```python
from build123d import *

# Parameters (mm, degrees)
SKETCH1_R           = 3
SKETCH1_R_2         = 1.6
BOSS_EXTRUDE1_DEPTH = 2.2
SKETCH1_3_R         = 1.6
BOSS_EXTRUDE2_DEPTH = 1
SKETCH5_R           = 1.5
BOSS_EXTRUDE3_DEPTH = 1
SKETCH6_R           = 2
BOSS_EXTRUDE4_DEPTH = 1
SKETCH8_R           = 1.5
BOSS_EXTRUDE5_DEPTH = 3
SKETCH10_R          = 2
BOSS_EXTRUDE6_DEPTH = 1


with BuildPart() as part:
    # Sketch1 → Boss-Extrude1 (new body)
    with BuildSketch(Plane(origin=(0, 0, 0), x_dir=(1, 0, 0), z_dir=(0, 1, 0))):
        with Locations((-0.522013312, 0.511138034)):
            Circle(SKETCH1_R)
        with Locations((-0.522013312, 0.511138034)):
            Circle(SKETCH1_R_2, mode=Mode.SUBTRACT)
    extrude(amount=BOSS_EXTRUDE1_DEPTH)

    # Sketch1_3 → Boss-Extrude2 (add)
    with BuildSketch(Plane(origin=(0, 0, 0), x_dir=(1, 0, 0), z_dir=(0, 1, 0))):
        with Locations((-0.522013312, 0.511138034)):
            Circle(SKETCH1_3_R)
    extrude(amount=BOSS_EXTRUDE2_DEPTH)

    # Sketch5 → Boss-Extrude3 (add)
    with BuildSketch(Plane.XZ):
        with Locations((-0.522013312, -0.511138034)):
            Circle(SKETCH5_R)
    extrude(amount=BOSS_EXTRUDE3_DEPTH)

    # Sketch6 → Boss-Extrude4 (add)
    with BuildSketch(Plane.XZ.offset(1)):
        with Locations((-0.522013312, -0.511138034)):
            Circle(SKETCH6_R)
    extrude(amount=BOSS_EXTRUDE4_DEPTH)

    # Sketch8 → Boss-Extrude5 (add)
    with BuildSketch(Plane(origin=(0, -2, 0), x_dir=(-1, 0, 0), z_dir=(0, -1, 0))):
        with Locations((0.522013312, 0.511138034)):
            Circle(SKETCH8_R)
    extrude(amount=BOSS_EXTRUDE5_DEPTH)

    # Sketch10 → Boss-Extrude6 (add)
    with BuildSketch(Plane.XZ.offset(5)):
        with Locations((-0.522013312, -0.511138034)):
            Circle(SKETCH10_R)
    extrude(amount=-BOSS_EXTRUDE6_DEPTH)


solid = part.part
```
Verification items for the finished model (mm, model axes). A direction names the side the tool comes from. Coordinates: 2 decimals unless noted, no trailing zeros. Write each loop counter-clockwise with the first axis right and the second up, starting at its lowest first coordinate (ties: lowest second). Pieces come first, ordered by that corner, then holes. Notation, with made-up numbers: M 89.5,5 L 141.5,5 A24 cw 141.5,34 Z; hole C 72,27.5 d6. An arc over 180 degrees is marked long. Answer as a JSON object with one key per item and string values. Group by question number.
(1) Cross-section at A-A, the plane z = 1.3. Record the cut outline in (x, y), and give its area (3 significant figures).
(2) Tool access check on faces 1 (the face through (-1, 1, -1)), 2 (the face through (0.91, -0.49, -0.06)), 3 (the face through (1.325, -1.493, -1.277)). Record the directions out of +Z, -Z, +X, -X, +Y, -Y that give a thin tool (end or side, any length) a straight path to the whole face; none if there is none.
(3) Gauge pin test, flat ends, axial feed: pin 1 (1.5 mm diameter, centred on y = -1.5, z = 0.5, fed in from -X); pin 2 (1.5 mm diameter, centred on x = -2, z = -0.5, fed in from +Y); pin 3 (1.5 mm diameter, centred on x = 1.5, z = 2, fed in from -Y); pin 4 (1 mm diameter, centred on x = 0, z = -1, fed in from +Y). Record the tip position at first contact, or that the pin passes through.
(4) Material ranges on line 1 (Y direction, x = -0.8, z = -0.15); line 2 (Z direction, x = -0.5, y = 1.75); line 3 (Y direction, x = -3.15, z = -1), recorded low to high.
(5) Cross-section at C-C, the plane z = 0.2. Record the cut outline in (x, y), and give its area (3 significant figures).
(6) Cross-section at B-B, the plane x = -2.4. Record the cut outline in (y, z).
(7) Release check for a two-part mould opening along X. For faces 4 (the face through (1, 0, 1)), 5 (the face through (-0.197, -2.986, 0.953)), 6 (the face through (1, 2, -1)) record: +X half, -X half, draft (parallel to the pull), parting line (faces both ways), or undercut.
(8) Cross-section at D-D, the plane x = 0.8. Record the cut outline in (y, z), and give its area (3 significant figures).
Reply:
{
 "1": {"outline": "M -2.91,0 L 1.87,0 L 1.87,2.2 L -2.91,2.2 Z; M -1.37,-5 L 0.33,-5 L 0.33,-4 L -1.37,-4 Z; M -1.37,-2 L 0.33,-2 L 0.33,-1 L -1.37,-1 Z", "area": "13.9 mm²"},
 "2": {"face 1": "+Y", "face 2": "none", "face 3": "-Y"},
 "3": {"pin 1": "x = -2.5", "pin 2": "y = 2.2", "pin 3": "y = 0", "pin 4": "y = 1"},
 "4": {"line 1": "-5 to 1", "line 2": "-3.51 to -2.11, 1.09 to 2.49", "line 3": "0 to 2.2"},
 "5": {"outline": "M -3.44,0 L -1.84,0 L -1.84,-1 L -2.39,-1 L -2.39,-2 L -1.84,-2 L -1.84,-4 L -2.39,-4 L -2.39,-5 L 1.35,-5 L 1.35,-4 L 0.8,-4 L 0.8,-2 L 1.35,-2 L 1.35,-1 L 0.8,-1 L 0.8,0 L 2.39,0 L 2.39,2.2 L 0.91,2.2 L 0.91,1 L -1.96,1 L -1.96,2.2 L -3.44,2.2 Z", "area": "24.8 mm²"},
 "6": {"outline": "M -5,-1.2 L -4,-1.2 L -4,0.18 L -5,0.18 Z; M -2,-1.2 L -1,-1.2 L -1,0.18 L -2,0.18 Z; M 0,-2.85 L 2.2,-2.85 L 2.2,1.83 L 0,1.83 Z"},
 "7": {"face 4": "draft", "face 5": "parting line", "face 6": "undercut"},
 "8": {"outline": "M -5,-2.01 L -4,-2.01 L -4,-1.22 L -2,-1.22 L -2,-2.01 L -1,-2.01 L -1,-1.22 L 0,-1.22 L 0,-3.2 L 2.2,-3.2 L 2.2,-1.41 L 1,-1.41 L 1,0.39 L 2.2,0.39 L 2.2,2.18 L 0,2.18 L 0,0.2 L -1,0.2 L -1,0.99 L -2,0.99 L -2,0.2 L -4,0.2 L -4,0.99 L -5,0.99 Z", "area": "19.9 mm²"}
}
